The model under review builds one solid part; all positions refer to its coordinate system, in mm. Round coordinates to 2 decimals unless told otherwise and drop trailing zeros. Write each loop counter-clockwise with the first axis right and the second up, starting at its lowest first coordinate (ties: lowest second). Pieces come first, ordered by that corner, then holes. Notation, with made-up numbers: (19, 46) - (67, 46) arc R17 ccw to (67, 54) - close; hole circle Ø3 at (14.5, 8.25). An arc over 180 degrees is marked (long way). Return JSON: item names as keys, results as strings.
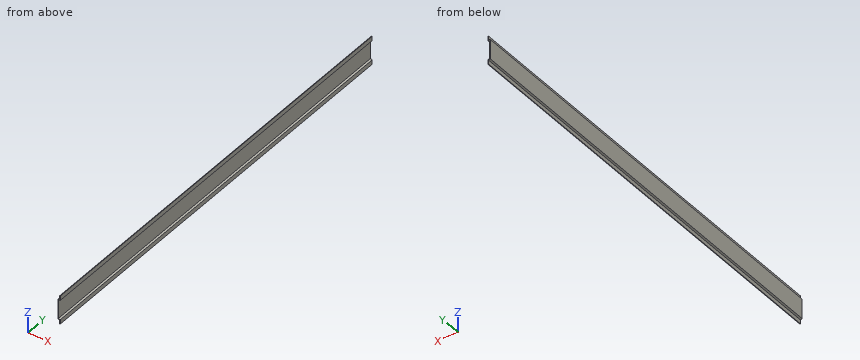
Autodesk Inventor part; units mm, degrees
ref_plane "YZ Plane" through (0, 0, 0) normal (1, 0, 0) x (0, 1, 0)
ref_plane "XZ Plane" through (0, 0, 0) normal (0, 1, 0) x (-1, 0, 0)
ref_plane "XY Plane" through (0, 0, 0) normal (0, 0, 1) x (1, 0, 0)
sketch "Skizze1" plane through (0, 0, 0) normal (0, 1, 0) x (-1, 0, 0)
  line L0 (0, 0) -> (1.15, 0) construction
  line L1 (1.15, 0) -> (1.15, -13) construction
  line L2 (1.15, -13) -> (0, -13) construction
  line L3 (0, -13) -> (0, 0) construction
  line L4 (0, -6.5) -> (1.15, -6.5) construction
  line L5 (0.575, -1.85) -> (0.575, -11.15) construction
  line L6 (0.3, -1.7763) -> (1.15, -2.0041) construction
  line L7 (0.85, -2.2343) -> (0, -2.0065) construction
  line L8 (0.3, 0) -> (0.3, -1.7763)
  line L9 (0.3, -11.2237) -> (1.15, -10.9959) construction
  line L10 (0, -10.9935) -> (0.85, -10.7657) construction
  line L11 (0.3, -11.2237) -> (0.3, -13)
  line L12 (0.85, -2.2343) -> (0.85, -10.7657)
  line L13 (0, 0) -> (0.3, 0)
  line L14 (0.3, -1.7763) -> (1.15, -2.0041)
  line L15 (1.15, -10.9959) -> (0.3, -11.2237)
  line L16 (0.3, -13) -> (0, -13)
  line L17 (0, -10.9935) -> (0.85, -10.7657)
  line L18 (0.85, -2.2343) -> (0, -2.0065)
  line L19 (1.15, -2.0041) -> (1.15, -10.9959)
  line L20 (0, -2.0065) -> (0, 0)
  line L21 (0, -10.9935) -> (0, -13)
  point P0 (0.575, -6.5)
  dimension "d0" = 1.15
  dimension "d1" = 13
  dimension "d4" = 9.3
  dimension "d7" = 75
  dimension "d8" = 0.3
  dimension "d9" = 0.3
  dimension "d10" = 75
  dimension "d11" = 0.3
  dimension "d12" = 0.3
extrude "Extrusion1" add sketch "Skizze1" along normal blind 200
equation "\"Biegeradius\" = Stärke"
equation "\"BreiteBiegungsfreistellung\" = Stärke"
equation "\"TiefeBiegungsfreistellung\" = 0.5 * Stärke"
equation "\"GrößeEckenfreistellung\" = 4 * Stärke"
equation "\"MinimalRest\" = 2 * Stärke"
equation "\"Übergangsradius\" = Biegeradius"
equation "\"JacobiRadiusGröße\" = Biegeradius"
equation "\"Abstandsgröße\" = Stärke"
properties part number "Koffer_ankerschiene_2m"
(1) Add section B-B (x = -0.55). Write out the cut boundary in (y, z).
Filled in:
{"outline": "(0, -11.16) - (200, -11.16) - (200, -10.85) - (0, -10.85) - close; (0, -2.15) - (200, -2.15) - (200, -1.84) - (0, -1.84) - close"}
(2) Add section A-A (y = 130). Write out the cut boundary in (x, z).
Filled in:
{"outline": "(-1.15, -11) - (-0.3, -11.22) - (-0.3, -13) - (0, -13) - (0, -10.99) - (-0.85, -10.77) - (-0.85, -2.23) - (0, -2.01) - (0, 0) - (-0.3, 0) - (-0.3, -1.78) - (-1.15, -2) - close"}
(3) Wall thickness on line 1 (Z direction, x = -0.1, y = 52); line 2 (X direction, y = 102, z = -12); line 3 (Z direction, x = -0.55, y = 9): over which ranges is each line inside the solid? List them lowest first.
Filled in:
{"line 1": "z = -13 to -10.97, -2.03 to 0", "line 2": "x = -0.3 to 0", "line 3": "z = -11.16 to -10.85, -2.15 to -1.84"}
(4) Add section C-C (z = -8). Write out the cut boundary in (x, y).
Filled in:
{"outline": "(-1.15, 0) - (-0.85, 0) - (-0.85, 200) - (-1.15, 200) - close"}
(5) Clearance check with flat-ended pins moving along their axes: pin 1 Ø7 at (y, z) = (119.5, -6.5) entering from +X; pin 2 Ø0.9 at (y, z) = (136, -12) entering from -X. State where each tip first meets the part, or that it passes through.
Filled in:
{"pin 1": "stops at x = -0.85", "pin 2": "stops at x = -0.3"}
